Autodesk Inventor part; units mm, degrees
ref_plane "YZ Plane" through (0, 0, 0) normal (1, 0, 0) x (0, 1, 0)
ref_plane "XZ Plane" through (0, 0, 0) normal (0, 1, 0) x (-1, 0, 0)
ref_plane "XY Plane" through (0, 0, 0) normal (0, 0, 1) x (1, 0, 0)
sketch "Sketch1" plane through (0, 0, 0) normal (0, 0, 1) x (1, 0, 0)
  line L0 (-13, 0) -> (13, 0)
  line L1 (13, 0) -> (12.25, 13)
  line L2 (12.25, 13) -> (14.2533, 13)
  line L3 (15, -2) -> (-15, -2)
  line L4 (-14.2533, 13) -> (-12.25, 13)
  line L5 (-12.25, 13) -> (-13, 0)
  line L6 (-15, -2) -> (-15, 0.0576)
  line L7 (-15, 0.0576) -> (-14.2533, 13)
  line L8 (15, -2) -> (15, 0.0576)
  line L9 (15, 0.0576) -> (14.2533, 13)
  point P0 (0, 0)
  point P1 (0, 0)
  point P2 (0, -2)
  dimension "d0" = 24.5
  dimension "d2" = 2
  dimension "d4" = 26
  dimension "d5" = 13
  dimension "d27" = 2
  dimension "d28" = 2
extrude "Extrusion1" add sketch "Sketch1" along normal blind 50
sketch "Sketch2" plane through (-15, -2, 0) normal (0, -1, 0) x (1, 0, 0)
  line L0 (0, 50) -> (30, 50)
  line L1 (0, 0) -> (0, 50)
  line L2 (15, 50) -> (-6.1309, 95.3154)
  line L3 (-18.4518, 89.5701) -> (6.19, 101.0607)
  line L4 (6.19, 101.0607) -> (27.3209, 55.7453)
  line L5 (27.3209, 55.7453) -> (2.6791, 44.2547)
  line L6 (2.6791, 44.2547) -> (-18.4518, 89.5701)
  line L7 (30, 50) -> (27.3209, 55.7453)
  point P0 (15, 0)
  dimension "d8" = 25
  dimension "d13" = 50
extrude "Extrusion2" add sketch "Sketch2" against normal up to surface (2 mm away)
sketch "Sketch3" plane through (-15, -2, 0) normal (0, -1, 0) x (1, 0, 0)
  line L0 (30, 0) -> (30, 50)
  line L1 (6.19, 101.0607) -> (-18.4518, 89.5701)
  line L2 (-18.4518, 89.5701) -> (0, 50)
  line L3 (-13.5341, 86.3464) -> (-12.6888, 84.5337)
  line L4 (-12.6888, 84.5337) -> (6.3436, 93.4087)
  line L5 (6.3436, 93.4087) -> (5.4984, 95.2213)
  line L6 (5.4984, 95.2213) -> (-13.5341, 86.3464)
  line L7 (-6.1309, 95.3154) -> (30, 17.8324) construction
  point P0 (30.2374, 50)
  point P1 (15, 0)
  point P2 (-4.0178, 90.7839)
  dimension "d17" = 21
  dimension "d19" = 5
  dimension "d20" = 2
extrude "Extrusion3" cut sketch "Sketch3" against normal through all
pattern_linear "Rectangular Pattern1" count 2 spacing 15 along (0.4226, 0, -0.9063) of "Extrusion3"
fillet "Fillet1" radius 5 2 edges at (-33.4518, -1, 89.5701) (-8.81, -1, 101.0607)
properties part number "tow ribbon management"
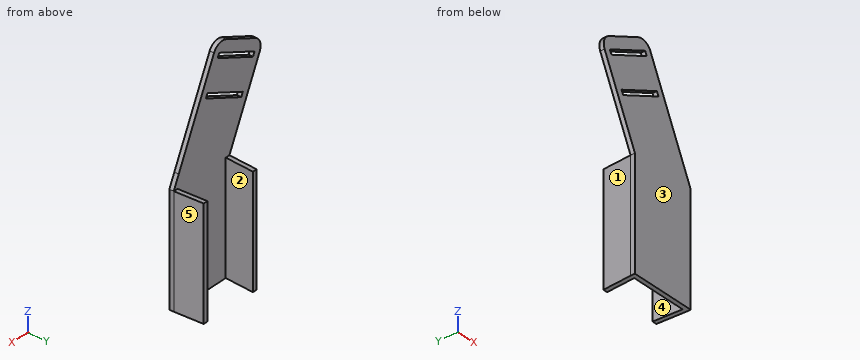
Read the model definition and answer for the solid it produces. Units are mm, in the model's axes. Face numbers are marked on the shaded views. A direction names the side the tool comes from. Coordinates: 2 decimals unless noted, no trailing zeros. Loops run counter-clockwise (first coordinate to the right, second up) from the corner with the lowest first, then second, coordinate; pieces in that order, holes last. Notation, with made-up numbers: (-35, 17.25) -> (-8, 17.25) arc R13 cw to (-8, 38.25) -> close; hole circle Ø4 at (-13, -2.5). An arc over 180 degrees is marked (long way). Answer in a Markdown table with one row per item.
Item 1: For a pull along Y with two mould halves and no side action, classify the marked faces 3, 4 and 5 as released by +Y, released by -Y, zero draft, split by the parting line, or undercut.
Returned:
| item | result |
|---|---|
| face 3 | released by -Y |
| face 4 | undercut |
| face 5 | released by +Y |
Item 2: A cutting plane is placed at B-B on y = 5.25. Determine the outline of the cut face in (x, z), plus the area to 3 significant figures.
Returned:
| item | result |
|---|---|
| outline | (-14.7, 0) -> (-12.7, 0) -> (-12.7, 50) -> (-14.7, 50) -> close; (12.7, 0) -> (14.7, 0) -> (14.7, 50) -> (12.7, 50) -> close |
| area | 200 mm^2 |
Item 3: A cutting plane is placed at C-C on z = 20. Determine the outline of the cut face in (x, y), plus the area to 3 significant figures.
Returned:
| item | result |
|---|---|
| outline | (-15, -2) -> (15, -2) -> (15, 0.06) -> (14.25, 13) -> (12.25, 13) -> (13, 0) -> (-13, 0) -> (-12.25, 13) -> (-14.25, 13) -> (-15, 0.06) -> close |
| area | 112 mm^2 |
Item 4: Each of these flat-tipped pins is pushed along its axis until it touches: P1, Ø1.4, axis at x = -14, y = 4, coming from the +Z side; P2, Ø1.5, axis at y = 7, z = 22, coming from the -X side; P3, Ø1, axis at y = -0.5, z = 13.5, coming from the -X side. Where does it stop, or does it pass through?
Returned:
| item | result |
|---|---|
| P1 | stops at z = 50 |
| P2 | stops at x = -14.64 |
| P3 | stops at x = -15 |
Item 5: A cutting plane is placed at A-A on x = -23.5. Determine the outline of the cut face in (y, z), plus the area to 3 significant figures.
Returned:
| item | result |
|---|---|
| outline | (-2, 68.23) -> (0, 68.23) -> (0, 86.49) -> (-2, 86.49) -> close; (-2, 88.69) -> (0, 88.69) -> (0, 94.21) -> (-2, 94.21) -> close |
| area | 47.6 mm^2 |
Item 6: Straight lines are drawn through the part: line 1 along X through (y, z) = (0.25, 29); line 2 along X through (y, z) = (9.25, 44); line 3 along Y through (x, z) = (5, 27.5). For each, find the intervals that lie inside material, in ascending order. Write a range as [from, to].
Returned:
| item | result |
|---|---|
| line 1 | x = [-14.99, -12.99], [12.99, 14.99] |
| line 2 | x = [-14.47, -12.47], [12.47, 14.47] |
| line 3 | y = [-2, 0] |
Item 7: A cutting plane is placed at D-D on x = 10. Determine the outline of the cut face in (y, z), plus the area to 3 significant figures.
Returned:
| item | result |
|---|---|
| outline | (-2, 0) -> (0, 0) -> (0, 60.72) -> (-2, 60.72) -> close |
| area | 121 mm^2 |
Item 8: For the marked faces 1 and 2, determine the directions among +Z, -Z, +X, -X, +Y, -Y from which every point of the face is accessible in a straight line to the end or side of a thin tool.
Returned:
| item | result |
|---|---|
| face 1 | +Z, -Z, -X, +Y |
| face 2 | +Z, -Z |
